```python
from build123d import *

# Parameters (mm, degrees)
SKETCH_1_R          = 4
EXTRUDE_1_DEPTH     = 8
SKETCH_2_R          = 2
EXTRUDE_2_DEPTH     = 3
CHAMFER_1_SIZE      = 1
FILLET_1_R          = 0.2
CUT_EXTRUDE_START   = -1
SKETCH_3_R          = 2.5
SKETCH_3_R_2        = 2
CUT_EXTRUDE_1_DEPTH = 1
FILLET_2_R          = 0.5


with BuildPart() as part:
    # 스케치1 → 보스-돌출1 (new body)
    with BuildSketch(Plane.XY):
        with BuildLine():
            Line((18.503045264, 25.710400876), (16.774192381, 12.269481729))
            ThreePointArc((16.774192381, 12.269481729), (16.649873032, 11.899636309), (16.393483216, 11.605518651))
            Line((16.393483216, 11.605518651), (6.818985785, 4.213374054))
            ThreePointArc((6.818985785, 4.213374054), (6.562595969, 3.919256395), (6.43827662, 3.549410976))
            Line((6.43827662, 3.549410976), (5.036897025, -7.345576114))
            ThreePointArc((5.036897025, -7.345576114), (4.885123304, -7.67333808), (4.572690124, -7.854580118))
            Line((4.572690124, -7.854580118), (-8.955561464, -10.878611884))
            ThreePointArc((-8.955561464, -10.878611884), (-9.059146158, -10.892441175), (-9.163559205, -10.888087594))
            ThreePointArc((-9.163559205, -10.888087594), (-9.247925369, -10.873458379), (-9.330730781, -10.851665551))
            Line((-9.330730781, -10.851665551), (-22.39641752, -6.807524417))
            ThreePointArc((-22.39641752, -6.807524417), (-22.542578492, -6.774052023), (-22.692101248, -6.762810308))
            Line((-22.692101248, -6.762810308), (-24.7735417, -6.762810308))
            ThreePointArc((-24.7735417, -6.762810308), (-25.480648481, -6.469917089), (-25.7735417, -5.762810308))
            Line((-25.7735417, -5.762810308), (-25.7735417, -1.895501216))
            ThreePointArc((-25.7735417, -1.895501216), (-25.62709509, -1.541947825), (-25.2735417, -1.395501216))
            Line((-25.2735417, -1.395501216), (-13.092668434, -1.395501216))
            Line((-13.092668434, -1.395501216), (-13.092668434, -2.589456262))
            Line((-13.092668434, -2.589456262), (-6.869177412, -2.589456262))
            ThreePointArc((-6.869177412, -2.589456262), (-6.474967763, -2.441782198), (-6.274806584, -2.071452104))
            Line((-6.274806584, -2.071452104), (-5.245859717, 5.387170068))
            ThreePointArc((-5.245859717, 5.387170068), (-5.205979224, 5.525201179), (-5.128493011, 5.646192616))
            Line((-5.128493011, 5.646192616), (6.347898488, 18.896175834))
            ThreePointArc((6.347898488, 18.896175834), (6.453984658, 19.043922748), (6.53155388, 19.208441568))
            Line((6.53155388, 19.208441568), (9.369909955, 26.995955233))
            ThreePointArc((9.369909955, 26.995955233), (9.579752789, 27.251863138), (9.903467507, 27.320650143))
            Line((9.903467507, 27.320650143), (18.070918344, 26.270102873))
            ThreePointArc((18.070918344, 26.270102873), (18.402899883, 26.07974829), (18.503045264, 25.710400876))
        make_face()
        Circle(SKETCH_1_R, mode=Mode.SUBTRACT)
    extrude(amount=EXTRUDE_1_DEPTH)

    # 스케치2 → 보스-돌출2 (add)
    with BuildSketch(Plane(origin=(3.618137143, 28.129107616, 0), x_dir=(0.9918289166876348, -0.1275750760228385, 0), z_dir=(0.1275750760228385, 0.9918289166876348, 0))):
        with Locations((10.454480212, -4)):
            Circle(SKETCH_2_R)
    extrude(amount=EXTRUDE_2_DEPTH)

    # 모따기1
    chamfer_1_edges = [part.edges().sort_by_distance(p)[0] for p in [
        (12.38626032, 30.02601341, 4),
    ]]
    chamfer(chamfer_1_edges, length=CHAMFER_1_SIZE)

    # 필렛1
    fillet_1_edges = [part.edges().sort_by_distance(p)[0] for p in [
        (-4, 0, 0),
        (-4, 0, 8),
    ]]
    fillet(fillet_1_edges, radius=FILLET_1_R)

    # 스케치3 → 컷-돌출1 (cut)
    with BuildSketch(Plane(origin=(3.618137143, 28.129107616, 0), x_dir=(0.9918289166876348, -0.1275750760228385, 0), z_dir=(0.1275750760228385, 0.9918289166876348, 0)).offset(CUT_EXTRUDE_START)):
        with Locations(Location((10.454480212, -4, 0), (0, 0, 180))):
            Circle(SKETCH_3_R)
        with Locations(Location((10.454480212, -4, 0), (0, 0, 180))):
            Circle(SKETCH_3_R_2, mode=Mode.SUBTRACT)
    extrude(amount=CUT_EXTRUDE_1_DEPTH, mode=Mode.SUBTRACT)

    # 필렛2
    fillet_2_edges = [part.edges().sort_by_distance(p)[0] for p in [
        (6.562595969, 3.919256395, 8),
        (11.606234501, 7.909446352, 8),
        (16.649873032, 11.899636309, 8),
        (17.638618823, 18.989941303, 8),
        (18.402899883, 26.07974829, 8),
        (-2.19143567, -9.366596001, 0),
        (-9.059146158, -10.892441175, 0),
        (-9.247925369, -10.873458379, 0),
        (-15.86357415, -8.829594984, 0),
        (-22.542578492, -6.774052023, 0),
        (-23.732821474, -6.762810308, 0),
        (13.987192925, 26.795376508, 8),
        (-25.480648481, -6.469917089, 0),
        (-25.7735417, -3.829155762, 0),
        (-25.62709509, -1.541947825, 0),
        (-19.183105067, -1.395501216, 0),
        (-9.980922923, -2.589456262, 0),
        (-6.474967763, -2.441782198, 0),
        (9.579752789, 27.251863138, 8),
        (-5.76033315, 1.657858982, 0),
        (-5.205979224, 5.525201179, 0),
        (0.609702738, 12.271184225, 0),
        (6.453984658, 19.043922748, 0),
        (7.950731917, 23.102198401, 0),
        (9.579752789, 27.251863138, 0),
        (13.987192925, 26.795376508, 0),
        (18.402899883, 26.07974829, 0),
        (7.950731917, 23.102198401, 8),
        (17.638618823, 18.989941303, 0),
        (16.649873032, 11.899636309, 0),
        (11.606234501, 7.909446352, 0),
        (6.562595969, 3.919256395, 0),
        (5.737586822, -1.898082569, 0),
        (4.885123304, -7.67333808, 0),
        (6.453984658, 19.043922748, 8),
        (0.609702738, 12.271184225, 8),
        (4.885123304, -7.67333808, 8),
        (-5.205979224, 5.525201179, 8),
        (-5.76033315, 1.657858982, 8),
        (-6.474967763, -2.441782198, 8),
        (-9.980922923, -2.589456262, 8),
        (-19.183105067, -1.395501216, 8),
        (-25.62709509, -1.541947825, 8),
        (-25.7735417, -3.829155762, 8),
        (-25.480648481, -6.469917089, 8),
        (-23.732821474, -6.762810308, 8),
        (5.737586822, -1.898082569, 8),
        (-22.542578492, -6.774052023, 8),
        (-15.86357415, -8.829594984, 8),
        (-9.247925369, -10.873458379, 8),
        (-9.059146158, -10.892441175, 8),
        (-2.19143567, -9.366596001, 8),
    ]]
    fillet(fillet_2_edges, radius=FILLET_2_R)


solid = part.part
```
Build history of the part. All positions in model axes, mm. A direction names the side the tool comes from. Coordinates: 2 decimals unless noted, no trailing zeros. Order: outer loops, then holes, each group sorted by start corner. A loop starts at its lowest first (then second) coordinate and runs counter-clockwise, first axis right, second up.
Item 1: Tool access for faces 4 (the flat face through (5.747, -1.822, 3.951)), 5 (the flat face through (-19, -1.396, 4)): list every direction of +Z, -Z, +X, -X, +Y, -Y with a clear straight run to the whole face (end or side of a thin tool).
Filled in:
face 4: +Z, -Z, +X, -Y
face 5: +Z, -Z, -X, +Y
Item 2: Drill centre lines: L1, parallel to X at y = 3.5, z = 2; L2, parallel to Y at x = -5, z = 5; L3, parallel to X at y = 19, z = 7. Where is each one in solid material? Low to high.
Filled in:
L1: x = -5.51 to -1.94, 1.94 to 6.43
L2: y = -9.99 to 5.79
L3: x = 6.43 to 17.64
Item 3: Drop flat-ended pins along their axis: pin 1 Ø1 at (x, z) = (-23.5, 2.5) entering from -Y; pin 2 Ø2 at (y, z) = (3, 3) entering from -X; pin 3 Ø1.4 at (y, z) = (-2.5, 6) entering from +X. Give the stop position or say it passes through.
Filled in:
pin 1: stops at y = -6.76
pin 2: stops at x = -5.71
pin 3: stops at x = 5.75
Item 4: Saw through at A-A on z = 7. List the corners of the cut face in (x, y).
Filled in:
outline: (-25.77, -5.76) arc R1 ccw to (-24.77, -6.76) - (-22.69, -6.76) arc R1 cw to (-22.4, -6.81) - (-9.33, -10.85) arc R1 ccw to (-9.16, -10.89) arc R0.6 ccw to (-8.96, -10.88) - (4.57, -7.85) arc R0.6 ccw to (5.04, -7.35) - (6.44, 3.55) arc R1 cw to (6.82, 4.21) - (16.39, 11.61) arc R1 ccw to (16.77, 12.27) - (18.5, 25.71) arc R0.5 ccw to (18.07, 26.27) - (9.9, 27.32) arc R0.5 ccw to (9.37, 27) - (6.53, 19.21) arc R1 cw to (6.35, 18.9) - (-5.13, 5.65) arc R0.5 ccw to (-5.25, 5.39) - (-6.27, -2.07) arc R0.6 cw to (-6.87, -2.59) - (-13.09, -2.59) - (-13.09, -1.4) - (-25.27, -1.4) arc R0.5 ccw to (-25.77, -1.9) - close; hole circle Ø8 at (0, 0)
Item 5: Mould opens along Z. For faces 1 (the cylindrical face through (14.25, 26.25, 6.48)), 2 (the flat face through (0.53, 12.18, 3.95)), 3 (the cylindrical face through (11.45, 7.97, 7.85)) say: released by +Z, released by -Z, zero draft, split by the parting line, or undercut.
Filled in:
face 1: undercut
face 2: zero draft
face 3: released by +Z
